Could you check a few things on this model? Use its own coordinates, in mm. A direction names the side the tool comes from. Give positions to 0.01 mm unless a question says otherwise; leave off trailing zeros. Order: outer loops, then holes, each group sorted by start corner. A loop starts at its lowest first (then second) coordinate and runs counter-clockwise, first axis right, second up. Notation, with made-up numbers: M 11,53.25 L 66,53.25 A26 cw 66,79.25 Z; hole C 18.25,23.25 d3. An arc over 180 degrees is marked long. Use a Markdown table: item, result. Add a question column.
Item 1: For faces 4 (the face through (-97.7, -5, 2)), 5 (the face through (-1, 52.512, 3)), which set-ups out of +Z, -Z, +X, -X, +Y, -Y let a thin tool reach every point of the face, with its end or its side?
Item 2: Suppose I cut it at C-C on x = 45.5. Write out the boundary of the cut face in (y, z), plus the area to 3 significant figures.
Item 3: Suppose I cut it at A-A on z = 2.25. Write out the boundary of the cut face in (x, y).
Item 4: Suppose I cut it at B-B on y = -11. Write out the boundary of the cut face in (x, z).
Item 5: I'm going to push a flat-ended pin straight in: pin 1 Ø4 at (x, y) = (-41.5, -13.5) entering from +Z. Where does the tip first touch, or does it pass through?
Item 6: If we mould it in two halves opening along Y, with no side actions, what happens to faces 1 (the face through (-94.259, 54.148, 5.645)), 2 (the face through (97.7, -6, 2)), 3 (the face through (95.116, 54.987, 2.45))? For each: released by +Y, released by -Y, zero draft, split by the parting line, or undercut.
Item 7: If I drill on L1, parallel to X at y = 21, z = 5; L2, parallel to Y at x = 52.5, z = 1.25; L3, parallel to Z at x = 81.5, y = -5, over which ranges is the centre line in solid material (lowest first)? Write a range as from..to.
from build123d import *

# Parameters (mm, degrees)
F1_DEPTH = 5.3
F2_DEPTH = 6
F3_DEPTH = 1.2
F4_R     = 2.5


with BuildPart() as f1:
    # F0 (on Top) → F1 (new body)
    with BuildSketch(Plane.XY):
        with BuildLine():
            Line((88.64, 56.511587), (-88.64, 56.511587))
            ThreePointArc((-88.64, 56.511587), (-94.197859, 54.209447), (-96.5, 48.651587))
            Line((-96.5, 48.651587), (-96.5, -46.428413))
            ThreePointArc((-96.5, -46.428413), (-94.197859, -51.986272), (-88.64, -54.288413))
            Line((-88.64, -54.288413), (88.64, -54.288413))
            ThreePointArc((88.64, -54.288413), (94.197859, -51.986272), (96.5, -46.428413))
            Line((96.5, -46.428413), (96.5, 48.651587))
            ThreePointArc((96.5, 48.651587), (94.197859, 54.209447), (88.64, 56.511587))
        make_face()
        with BuildLine():
            ThreePointArc((-92.5, 48.651587), (-91.369432, 51.38102), (-88.64, 52.511587))
            Line((-88.64, 52.511587), (88.64, 52.511587))
            ThreePointArc((88.64, 52.511587), (91.369432, 51.38102), (92.5, 48.651587))
            Line((92.5, 48.651587), (92.5, -46.428413))
            ThreePointArc((92.5, -46.428413), (91.369432, -49.157845), (88.64, -50.288413))
            Line((88.64, -50.288413), (-88.64, -50.288413))
            ThreePointArc((-88.64, -50.288413), (-91.369432, -49.157845), (-92.5, -46.428413))
            Line((-92.5, -46.428413), (-92.5, 48.651587))
        make_face(mode=Mode.SUBTRACT)
    extrude(amount=F1_DEPTH)

    # F0 (on Top) → F2 (join)
    with BuildSketch(Plane.XY):
        with BuildLine():
            ThreePointArc((-88.64, 57.711587), (-95.046387, 55.057975), (-97.7, 48.651587))
            Line((-97.7, 48.651587), (-97.7, -46.428413))
            Line((-97.7, -46.428413), (-97.7, -62.288413))
            Line((-97.7, -62.288413), (97.7, -62.288413))
            Line((97.7, -62.288413), (97.7, -46.428413))
            Line((97.7, -46.428413), (97.7, 48.651587))
            ThreePointArc((97.7, 48.651587), (95.046387, 55.057975), (88.64, 57.711587))
            Line((88.64, 57.711587), (-88.64, 57.711587))
        make_face()
        with BuildLine():
            ThreePointArc((-96.5, 48.651587), (-94.197859, 54.209447), (-88.64, 56.511587))
            Line((-88.64, 56.511587), (88.64, 56.511587))
            ThreePointArc((88.64, 56.511587), (94.197859, 54.209447), (96.5, 48.651587))
            Line((96.5, 48.651587), (96.5, -46.428413))
            ThreePointArc((96.5, -46.428413), (94.197859, -51.986272), (88.64, -54.288413))
            Line((88.64, -54.288413), (-88.64, -54.288413))
            ThreePointArc((-88.64, -54.288413), (-94.197859, -51.986272), (-96.5, -46.428413))
            Line((-96.5, -46.428413), (-96.5, 48.651587))
        make_face(mode=Mode.SUBTRACT)
    extrude(amount=F2_DEPTH)

    # F0 (on Top) → F3 (join)
    with BuildSketch(Plane.XY):
        with BuildLine():
            ThreePointArc((-88.64, 57.711587), (-95.046387, 55.057975), (-97.7, 48.651587))
            Line((-97.7, 48.651587), (-97.7, -46.428413))
            Line((-97.7, -46.428413), (-97.7, -62.288413))
            Line((-97.7, -62.288413), (97.7, -62.288413))
            Line((97.7, -62.288413), (97.7, -46.428413))
            Line((97.7, -46.428413), (97.7, 48.651587))
            ThreePointArc((97.7, 48.651587), (95.046387, 55.057975), (88.64, 57.711587))
            Line((88.64, 57.711587), (-88.64, 57.711587))
        make_face()
        with BuildLine():
            ThreePointArc((-96.5, 48.651587), (-94.197859, 54.209447), (-88.64, 56.511587))
            Line((-88.64, 56.511587), (88.64, 56.511587))
            ThreePointArc((88.64, 56.511587), (94.197859, 54.209447), (96.5, 48.651587))
            Line((96.5, 48.651587), (96.5, -46.428413))
            ThreePointArc((96.5, -46.428413), (94.197859, -51.986272), (88.64, -54.288413))
            Line((88.64, -54.288413), (-88.64, -54.288413))
            ThreePointArc((-88.64, -54.288413), (-94.197859, -51.986272), (-96.5, -46.428413))
            Line((-96.5, -46.428413), (-96.5, 48.651587))
        make_face(mode=Mode.SUBTRACT)
        with BuildLine():
            Line((88.64, 56.511587), (-88.64, 56.511587))
            ThreePointArc((-88.64, 56.511587), (-94.197859, 54.209447), (-96.5, 48.651587))
            Line((-96.5, 48.651587), (-96.5, -46.428413))
            ThreePointArc((-96.5, -46.428413), (-94.197859, -51.986272), (-88.64, -54.288413))
            Line((-88.64, -54.288413), (88.64, -54.288413))
            ThreePointArc((88.64, -54.288413), (94.197859, -51.986272), (96.5, -46.428413))
            Line((96.5, -46.428413), (96.5, 48.651587))
            ThreePointArc((96.5, 48.651587), (94.197859, 54.209447), (88.64, 56.511587))
        make_face()
        with BuildLine():
            ThreePointArc((-92.5, 48.651587), (-91.369432, 51.38102), (-88.64, 52.511587))
            Line((-88.64, 52.511587), (88.64, 52.511587))
            ThreePointArc((88.64, 52.511587), (91.369432, 51.38102), (92.5, 48.651587))
            Line((92.5, 48.651587), (92.5, -46.428413))
            ThreePointArc((92.5, -46.428413), (91.369432, -49.157845), (88.64, -50.288413))
            Line((88.64, -50.288413), (-88.64, -50.288413))
            ThreePointArc((-88.64, -50.288413), (-91.369432, -49.157845), (-92.5, -46.428413))
            Line((-92.5, -46.428413), (-92.5, 48.651587))
        make_face(mode=Mode.SUBTRACT)
        with BuildLine():
            Line((88.64, 52.511587), (-88.64, 52.511587))
            ThreePointArc((-88.64, 52.511587), (-91.369432, 51.38102), (-92.5, 48.651587))
            Line((-92.5, 48.651587), (-92.5, -46.428413))
            ThreePointArc((-92.5, -46.428413), (-91.369432, -49.157845), (-88.64, -50.288413))
            Line((-88.64, -50.288413), (88.64, -50.288413))
            ThreePointArc((88.64, -50.288413), (91.369432, -49.157845), (92.5, -46.428413))
            Line((92.5, -46.428413), (92.5, 48.651587))
            ThreePointArc((92.5, 48.651587), (91.369432, 51.38102), (88.64, 52.511587))
        make_face()
    extrude(amount=-F3_DEPTH)

    # F4
    f4_edges = [f1.edges().sort_by_distance(p)[0] for p in [
        (97.7, -62.288413, 2.4),
        (-97.7, -62.288413, 2.4),
    ]]
    fillet(f4_edges, radius=F4_R)


solid = f1.part
Findings below:
| question | item | result |
|---|---|---|
| 1 | face 4 | +Z, -Z, -X, +Y, -Y |
| 1 | face 5 | +Z |
| 2 | outline | M -62.29,-1.2 L 57.71,-1.2 L 57.71,6 L 56.51,6 L 56.51,5.3 L 52.51,5.3 L 52.51,0 L -50.29,0 L -50.29,5.3 L -54.29,5.3 L -54.29,6 L -62.29,6 Z |
| 2 | area | 242 mm^2 |
| 3 | outline | M -97.7,-59.79 A2.5 ccw -95.2,-62.29 L 95.2,-62.29 A2.5 ccw 97.7,-59.79 L 97.7,48.65 A9.06 ccw 88.64,57.71 L -88.64,57.71 A9.06 ccw -97.7,48.65 Z; hole M -92.5,-46.43 A3.86 ccw -88.64,-50.29 L 88.64,-50.29 A3.86 ccw 92.5,-46.43 L 92.5,48.65 A3.86 ccw 88.64,52.51 L -88.64,52.51 A3.86 ccw -92.5,48.65 Z |
| 4 | outline | M -97.7,-1.2 L 97.7,-1.2 L 97.7,6 L 96.5,6 L 96.5,5.3 L 92.5,5.3 L 92.5,0 L -92.5,0 L -92.5,5.3 L -96.5,5.3 L -96.5,6 L -97.7,6 Z |
| 5 | pin 1 | stops at z = 0 |
| 6 | face 1 | undercut |
| 6 | face 2 | zero draft |
| 6 | face 3 | released by +Y |
| 7 | L1 | x = -97.7..-92.5, 92.5..97.7 |
| 7 | L2 | y = -62.29..-50.29, 52.51..57.71 |
| 7 | L3 | z = -1.2..0 |
